Could you check a few things on this model? Use its own coordinates, in mm. A direction names the side the tool comes from. Round coordinates to 2 decimals unless told otherwise and drop trailing zeros. Write each loop counter-clockwise with the first axis right and the second up, starting at its lowest first coordinate (ties: lowest second). Pieces come first, ordered by that corner, then holes. Notation, with made-up numbers: (78, 37.25) -> (105, 37.25) arc R10 ccw to (105, 47.25) -> close; hole circle Ø8 at (-9.75, -32). An arc over 180 degrees is marked (long way). Answer in a Markdown table with one row per item.
from build123d import *

# Parameters (mm, degrees)
F3_D = 18


with BuildPart() as f1:
    # F0 (on Front) → F1 (revolve)
    with BuildSketch(Plane.XZ):
        Polygon((10.919107, 50), (0, 20), (0, 0), (24, 0), (24, 10), (12, 10), (8, 10), (8, 13), (7, 13), (7, 19), (12, 19), (12, 50), align=None)
    revolve(axis=Axis((12, 0, 0), (-1, 0, 0)))

    # F3 (through all)
    with Locations(Plane(origin=(0, 0, 0), x_dir=(0, 1, 0), z_dir=(-1, 0, 0))):
        with Locations((0, 0)):
            Hole(F3_D / 2)


solid = f1.part
1) For pin 1 (10 mm diameter, centred on x = 10.5, z = -3.5, fed in from +Y); pin 2 (1.5 mm diameter, centred on y = -9.5, z = 32.5, fed in from -X); pin 3 (8 mm diameter, centred on y = -5, z = -26, fed in from -X), each with a flat end and sliding along its axis, tell me the tip position at first contact or that it passes through.
Findings:
| item | result |
|---|---|
| pin 1 | stops at y = 50 |
| pin 2 | stops at x = 4.77 |
| pin 3 | stops at x = 0.9 |
2) Imagine slicing it at A-A, the plane y = 0. Please give me the cut outline in (x, z).
Findings:
| item | result |
|---|---|
| outline | (0, -20) -> (10.92, -50) -> (12, -50) -> (12, -19) -> (7, -19) -> (7, -13) -> (8, -13) -> (8, -10) -> (24, -10) -> (24, -9) -> (0, -9) -> close; (0, 9) -> (24, 9) -> (24, 10) -> (8, 10) -> (8, 13) -> (7, 13) -> (7, 19) -> (12, 19) -> (12, 50) -> (10.92, 50) -> (0, 20) -> close |
3) Please list where these lines run through material, in increasing order: line 1 (X direction, y = 12.5, z = -12); line 2 (X direction, y = -14, z = -38); line 3 (Z direction, x = 11, y = 25).
Findings:
| item | result |
|---|---|
| line 1 | x = 0 to 7 |
| line 2 | x = 7.46 to 12 |
| line 3 | z = -43.3 to 43.3 |
4) Imagine slicing it at C-C, the plane x = 1.75. Please give me the cut outline in (y, z), plus the area to 3 significant figures.
Findings:
| item | result |
|---|---|
| outline | circle Ø49.62 at (0, 0); hole circle Ø18 at (0, 0) |
| area | 1,680 mm^2 |
5) For faces 4 (the face through (24, 2, 9)), 5 (the face through (7.493, -7.91, -10.316)), which set-ups out of +Z, -Z, +X, -X, +Y, -Y let a thin tool reach every point of the face, with its end or its side?
Findings:
| item | result |
|---|---|
| face 4 | +Z, -Z, +X, +Y, -Y |
| face 5 | +X |
6) Thinking about a two-plate mould opening in Y: for faces 1 (the face through (11.45, 15.02, 47.69)), 2 (the face through (12.168, 1.172, -8.923)), 3 (the face through (12, -22, 1)), which applies, +Y half, -Y half, draft (parallel to the pull), parting line (faces both ways), or undercut?
Findings:
| item | result |
|---|---|
| face 1 | parting line |
| face 2 | undercut |
| face 3 | draft |
